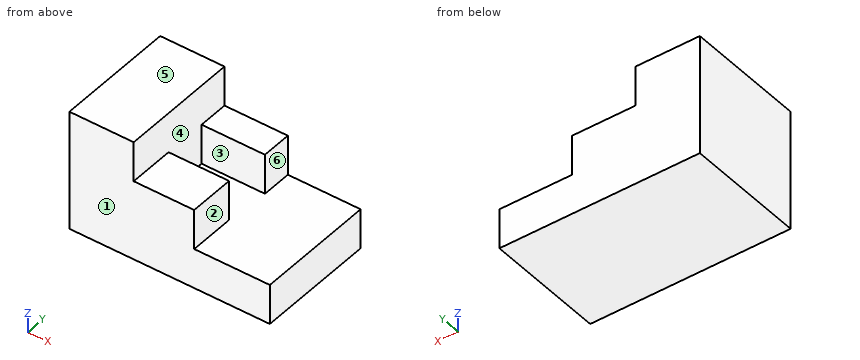
```python
from build123d import *

# Parameters (mm, degrees)
F0_W     = 127
F0_H     = 76.2
F1_DEPTH = 25.4
F2_W     = 40.7456940264
F2_H     = 76.2
F3_DEPTH = 50.8
F4_W     = 40.1406884193
F4_H     = 19.1947049409
F5_DEPTH = 25.4
F6_W     = 38.3402202278
F6_H     = 29.2502096802
F7_DEPTH = 25.4


with BuildPart() as f1:
    # F0 (on Top) → F1 (new body)
    with BuildSketch(Plane.XY):
        Rectangle(F0_W, F0_H)
    extrude(amount=F1_DEPTH)

    # F2 (on face) → F3 (join)
    with BuildSketch(Plane.XY.offset(25.4)):
        with Locations((-43.1271529868, 0)):
            Rectangle(F2_W, F2_H)
    extrude(amount=F3_DEPTH)

    # F4 (on face) → F5 (join)
    with BuildSketch(Plane.XY.offset(25.4)):
        with Locations((-2.683961764, 28.5026475295)):
            Rectangle(F4_W, F4_H)
    extrude(amount=F5_DEPTH)

    # F6 (on face) → F7 (join)
    with BuildSketch(Plane.XY.offset(25.4)):
        with Locations((-3.5841958597, -23.4748951599)):
            Rectangle(F6_W, F6_H)
    extrude(amount=F7_DEPTH)


solid = f1.part
```
Can you work these out from the model? Positions are in its coordinate system, mm. Face numbers are marked on the shaded views. A direction names the side the tool comes from. Give positions to 0.01 mm unless a question says otherwise; leave off trailing zeros. Loops run counter-clockwise (first coordinate to the right, second up) from the corner with the lowest first, then second, coordinate; pieces in that order, holes last. Notation, with made-up numbers: M -6,38 L 42,38 A29 cw 42,69 Z; hole C 87,76 d7. An arc over 180 degrees is marked long. Answer in a Markdown table with one row per item.
1. Suppose I cut it at D-D on y = 9. Write out the boundary of the cut face in (x, z).
Taken from the geometry:
| item | result |
|---|---|
| outline | M -63.5,0 L 63.5,0 L 63.5,25.4 L -22.75,25.4 L -22.75,76.2 L -63.5,76.2 Z |
2. Which directions (+Z, -Z, +X, -X, +Y, -Y) give clear straight access to the entire face, cutting with the end or side of a thin tool? Please do the marked faces 5 and 6.
Taken from the geometry:
| item | result |
|---|---|
| face 5 | +Z, +X, -X, +Y, -Y |
| face 6 | +Z, +X, +Y, -Y |
3. Thinking about a two-plate mould opening in Y: for the marked faces 1, 2, 3 and 4, which applies, released by +Y, released by -Y, zero draft, split by the parting line, or undercut?
Taken from the geometry:
| item | result |
|---|---|
| face 1 | released by -Y |
| face 2 | zero draft |
| face 3 | undercut |
| face 4 | undercut |
4. If I drill on line 1 along Y through (x, z) = (-6, 26); line 2 along Z through (x, y) = (-15, -15); line 3 along X through (y, z) = (-5, 52.5), over which ranges is the centre line in solid material (lowest first)?
Taken from the geometry:
| item | result |
|---|---|
| line 1 | y = -38.1 to -8.85, 18.91 to 38.1 |
| line 2 | z = 0 to 50.8 |
| line 3 | x = -63.5 to -22.75 |
5. Suppose I cut it at A-A on z = 30. Write out the boundary of the cut face in (x, y).
Taken from the geometry:
| item | result |
|---|---|
| outline | M -63.5,-38.1 L 15.59,-38.1 L 15.59,-8.85 L -22.75,-8.85 L -22.75,18.91 L 17.39,18.91 L 17.39,38.1 L -63.5,38.1 Z |
6. Suppose I cut it at B-B on y = 26. Write out the boundary of the cut face in (x, z), plus the area to 3 significant figures.
Taken from the geometry:
| item | result |
|---|---|
| outline | M -63.5,0 L 63.5,0 L 63.5,25.4 L 17.39,25.4 L 17.39,50.8 L -22.75,50.8 L -22.75,76.2 L -63.5,76.2 Z |
| area | 6,320 mm² |
7. For pin 1 Ø3 at (y, z) = (16.5, 42.5) entering from +X; pin 2 Ø23 at (x, y) = (26.5, -9) entering from +Z; pin 3 Ø15 at (y, z) = (-5.5, 39) entering from +X, each with a flat end and sliding along its axis, tell me the tip position at first contact or that it passes through.
Taken from the geometry:
| item | result |
|---|---|
| pin 1 | stops at x = -22.75 |
| pin 2 | stops at z = 50.8 |
| pin 3 | stops at x = 15.59 |
8. Suppose I cut it at C-C on x = 19. Write out the boundary of the cut face in (y, z), plus the area to 3 significant figures.
Taken from the geometry:
| item | result |
|---|---|
| outline | M -38.1,0 L 38.1,0 L 38.1,25.4 L -38.1,25.4 Z |
| area | 1,940 mm² |
